Autodesk Inventor part; units mm, degrees
ref_plane "YZ Plane" through (0, 0, 0) normal (1, 0, 0) x (0, 1, 0)
ref_plane "XZ Plane" through (0, 0, 0) normal (0, 1, 0) x (-1, 0, 0)
ref_plane "XY Plane" through (0, 0, 0) normal (0, 0, 1) x (1, 0, 0)
sketch "Sketch2" plane through (0, 0, 0) normal (0, 0, 1) x (1, 0, 0)
  line L0 (-75, -25) -> (75, -25)
  line L1 (75, -25) -> (75, 25)
  line L2 (75, 25) -> (-75, 25)
  line L3 (-75, 25) -> (-75, -25)
  line L4 (-75, -25) -> (75, 25) construction
  line L5 (75, -25) -> (-75, 25) construction
  point P0 (0, 0)
  dimension "d1" = 150
  dimension "d2" = 50
extrude "Extrusion1" add sketch "Sketch2" along normal mid plane 10
sketch "Sketch3" plane through (0, 0, 5) normal (0, 0, 1) x (1, 0, 0)
  line L0 (-75, 25) -> (-75, -25)
  line L1 (75, 25) -> (-75, 25)
  point P0 (0, 0)
  point P1 (-65, 0)
  dimension "d40" = 10
  dimension "d43" = 25
hole "Hole1" at (-65, 0, 5) direction (0, 0, -1) diameter 5.5 depth 14.2 tip angle 118 countersink diameter 10.4 countersink angle 90
sketch "Sketch4" plane through (0, 0, 5) normal (0, 0, 1) x (1, 0, 0)
  line L0 (-75, 25) -> (-75, -25)
  line L1 (75, 25) -> (-75, 25)
  point P0 (0, 0)
  point P1 (-45, 5)
  dimension "d41" = 30
  dimension "d42" = 20
hole "Hole2" at (-45, 5, 5) direction (0, 0, -1) diameter 6.6 depth 17.1 tip angle 118 countersink diameter 12.6 countersink angle 90
sketch "Sketch5" plane through (0, 0, 5) normal (0, 0, 1) x (1, 0, 0)
  line L0 (-75, 25) -> (-75, -25)
  line L1 (75, 25) -> (-75, 25)
  point P0 (0, 0)
  point P1 (-24, 10)
  dimension "d44" = 51
  dimension "d45" = 15
hole "Hole3" at (-24, 10, 5) direction (0, 0, -1) diameter 9 depth 22.2 tip angle 118 countersink diameter 17.3 countersink angle 90
sketch "Sketch6" plane through (0, 0, 5) normal (0, 0, 1) x (1, 0, 0)
  line L0 (-75, 25) -> (-75, -25)
  line L1 (75, 25) -> (-75, 25)
  point P0 (0, 0)
  point P1 (6, 5)
  dimension "d46" = 81
  dimension "d47" = 20
hole "Hole4" at (6, 5, 5) direction (0, 0, -1) diameter 6 depth 14.2 tip angle 118
sketch "Sketch7" plane through (0, 0, 5) normal (0, 0, 1) x (1, 0, 0)
  line L0 (-75, 25) -> (-75, -25)
  line L1 (75, 25) -> (-75, 25)
  point P0 (0, 0)
  point P1 (25, 10)
  dimension "d48" = 100
  dimension "d49" = 15
hole "Hole5" at (25, 10, 5) direction (0, 0, -1) diameter 10 depth 14.2 tip angle 118
pattern_linear "Rectangular Pattern1" count 3 spacing 10 along (0, -1, 0) of "Hole1" first direction both ways yes
mirror "Mirror1" about plane through (0, 0, 0) normal (0, 1, 0) of "Hole2"
mirror "Mirror2" about plane through (0, 0, 0) normal (0, 1, 0) of "Hole3"
pattern_linear "Rectangular Pattern2" count 3 spacing 10 along (0, -1, 0) of "Hole4"
mirror "Mirror3" about plane through (0, 0, 0) normal (0, 1, 0) of "Hole5"
properties part number "홀간 거리 확인 파트-13" material "SS400"
The listing builds one solid part. Answer for the finished solid, in the listing's coordinates (mm). Round coordinates to 2 decimals unless told otherwise and drop trailing zeros. Order: outer loops, then holes, each group sorted by start corner. A loop starts at its lowest first (then second) coordinate and runs counter-clockwise, first axis right, second up. Notation, with made-up numbers: (83, 72.5) -> (105, 72.5) arc R31 ccw to (105, 98.5) -> close; hole circle Ø4 at (86.25, -33.75). An arc over 180 degrees is marked (long way). One line per item, written item: value.
Item 1: For a pull along X with two mould halves and no side action, classify faces 1 (the conical face through (-66.11, -12.68, 2.7)), 2 (the flat face through (75, 0, 0)), 3 (the flat face through (-1, 0, -5)) as released by +X, released by -X, zero draft, split by the parting line, or undercut.
Taken from the geometry:
face 1: undercut
face 2: released by +X
face 3: zero draft
Item 2: Find section B-B, the plane x = 6. Give the vertices of the cut face in (y, z).
Taken from the geometry:
outline: (-25, -5) -> (-18, -5) -> (-18, 5) -> (-25, 5) -> close; (-12, -5) -> (-8, -5) -> (-8, 5) -> (-12, 5) -> close; (-2, -5) -> (2, -5) -> (2, 5) -> (-2, 5) -> close; (8, -5) -> (25, -5) -> (25, 5) -> (8, 5) -> close
Item 3: Find section C-C, the plane z = -2.5. State how many separate pieces and enclosed holes the cut face has, then the cut area to 3 significant figures.
Taken from the geometry:
separate pieces: 1
enclosed holes: 12
area: 6,990 mm2
Item 4: Straight lines are drawn through the part: L1, parallel to X at y = -10, z = -2.5; L2, parallel to Y at x = -24, z = -0.65; L3, parallel to Y at x = -65, z = -1.5. For each, find the intervals that lie inside material, in ascending order.
Taken from the geometry:
L1: x = -75 to -67.75, -62.25 to -28.5, -19.5 to 20, 30 to 75
L2: y = -25 to -14.5, -5.5 to 5.5, 14.5 to 25
L3: y = -25 to -12.75, -7.25 to -2.75, 2.75 to 7.25, 12.75 to 25
Item 5: Find section A-A, the plane x = 25. Give the vertices of the cut face in (y, z), then the cut area to 3 significant figures.
Taken from the geometry:
outline: (-25, -5) -> (-15, -5) -> (-15, 5) -> (-25, 5) -> close; (-5, -5) -> (5, -5) -> (5, 5) -> (-5, 5) -> close; (15, -5) -> (25, -5) -> (25, 5) -> (15, 5) -> close
area: 300 mm2
Item 6: Find section D-D, the plane x = -45. Give the vertices of the cut face in (y, z).
Taken from the geometry:
outline: (-25, -5) -> (-8.3, -5) -> (-8.3, 2) -> (-11.3, 5) -> (-25, 5) -> close; (-1.7, -5) -> (1.7, -5) -> (1.7, 2) -> (0, 3.7) -> (-1.7, 2) -> close; (8.3, -5) -> (25, -5) -> (25, 5) -> (11.3, 5) -> (8.3, 2) -> close
Item 7: Given P1, Ø3.5, axis at x = -65, y = 0, coming from the -Z side; P2, Ø10.5, axis at x = -24, y = -10, coming from the +Z side, each flat-ended and moving along its own axis, determine where each tip first touches the part or whether it passes through.
Taken from the geometry:
P1: passes through
P2: stops at z = 1.6
